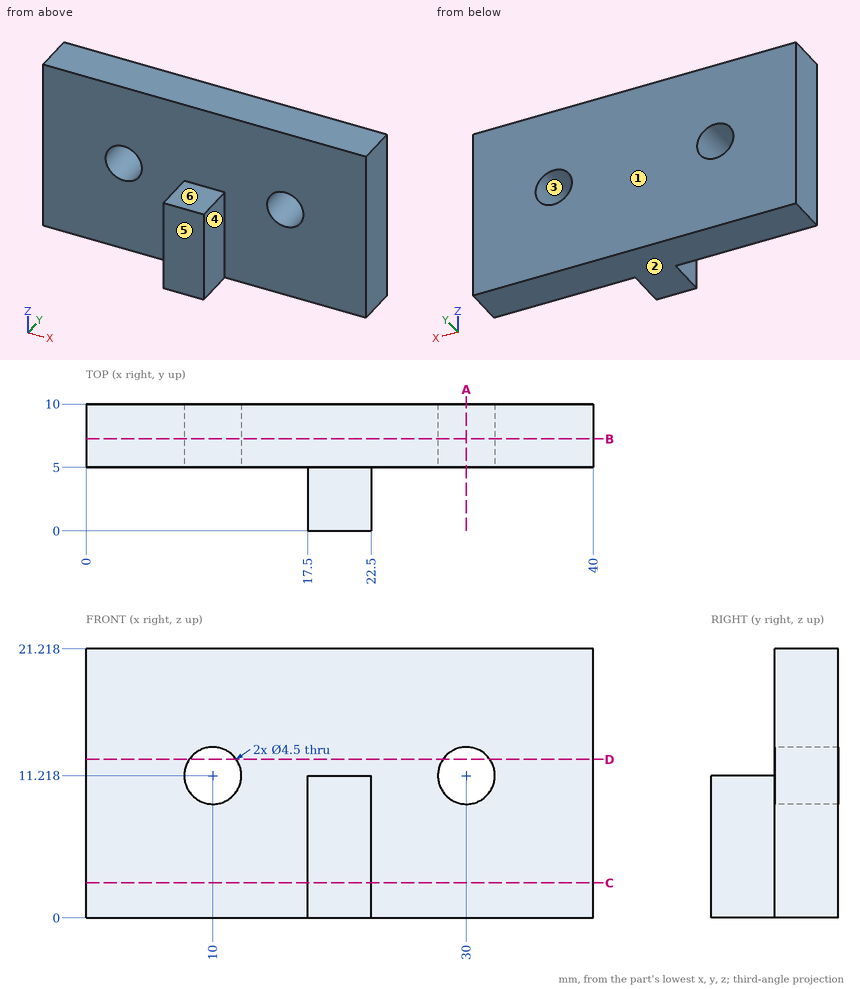
Geometry check sheet. Reference: drawing and pictorial views, mm from the part's lowest x, y, z. A direction names the side the tool comes from. Round coordinates to 2 decimals unless told otherwise and drop trailing zeros. Order: outer loops, then holes, each group sorted by start corner. A loop starts at its lowest first (then second) coordinate and runs counter-clockwise, first axis right, second up. Notation, with made-up numbers: (-36.75, 18.5) -> (-16.75, 18.5) arc R5 ccw to (-16.75, 23.5) -> close; hole circle Ø9 at (87.5, 22). An arc over 180 degrees is marked (long way). One line per item, written item: value. Start each with the question number.
Q1. Cross-section at B-B (y = 7.25). Record the boundary of the cut face in (x, z).
Q2. Cross-section at A-A (x = 30). Record the boundary of the cut face in (y, z), and give its area (3 significant figures).
Q3. Gauge pin test, flat ends, axial feed: pin 1 Ø2.5 at (y, z) = (2, 7.5) entering from +X; pin 2 Ø1.5 at (y, z) = (2, 4) entering from -X; pin 3 Ø1 at (x, z) = (6, 9) entering from -Y. Record the tip position at first contact, or that the pin passes through.
Q4. Cross-section at D-D (z = 12.5). Record the boundary of the cut face in (x, y), and give its area (3 significant figures).
Q5. Thickness scan on line 1 (Z direction, x = 10, y = 6.65); line 2 (X direction, y = 8.25, z = 12); line 3 (Y direction, x = 11, z = 2.25). Record the ranges inside material, lowest first.
Q6. Set-up check for the marked faces 4, 5 and 6: record each of +Z, -Z, +X, -X, +Y, -Y from which the full face is reachable in a straight line by a thin tool's end or side.
Q7. Cross-section at C-C (z = 2.75). Record the boundary of the cut face in (x, y), and give its area (3 significant figures).
Q8. Mould release check, pull along Z, two halves, no side actions. Record for the marked faces 1, 2 and 3: pulls with the +Z half, pulls with the -Z half, needs draft (parallel to the pull), parting line crosses it, or undercut.
Completed:
1. outline: (0, 0) -> (40, 0) -> (40, 21.22) -> (0, 21.22) -> close; hole circle Ø4.5 at (10, 11.22); hole circle Ø4.5 at (30, 11.22)
2. outline: (5, 0) -> (10, 0) -> (10, 8.97) -> (5, 8.97) -> close; (5, 13.47) -> (10, 13.47) -> (10, 21.22) -> (5, 21.22) -> close
2. area: 83.6 mm²
3. pin 1: stops at x = 22.5
3. pin 2: stops at x = 17.5
3. pin 3: stops at y = 5
4. outline: (0, 5) -> (8.15, 5) -> (8.15, 10) -> (0, 10) -> close; (11.85, 5) -> (28.15, 5) -> (28.15, 10) -> (11.85, 10) -> close; (31.85, 5) -> (40, 5) -> (40, 10) -> (31.85, 10) -> close
4. area: 163 mm²
5. line 1: z = 0 to 8.97, 13.47 to 21.22
5. line 2: x = 0 to 7.89, 12.11 to 27.89, 32.11 to 40
5. line 3: y = 5 to 10
6. face 4: +Z, -Z, +X, -Y
6. face 5: +Z, -Z, +X, -X, -Y
6. face 6: +Z, +X, -X, -Y
7. outline: (0, 5) -> (17.5, 5) -> (17.5, 0) -> (22.5, 0) -> (22.5, 5) -> (40, 5) -> (40, 10) -> (0, 10) -> close
7. area: 225 mm²
8. face 1: needs draft
8. face 2: pulls with the -Z half
8. face 3: undercut
